```python
from build123d import *

# Parameters (mm, degrees)
BOSS_EXTRUDE1_DEPTH = 3
BOSS_EXTRUDE5_DEPTH = 11.5
SKETCH7_W           = 32.25
SKETCH7_H           = 15
SKETCH7_R           = 3
BOSS_EXTRUDE6_DEPTH = 3.5
FILLET4_R           = 4
FILLET5_R           = 5
FILLET6_SIZE        = 5
FILLET6_SIZE_2      = 15
FILLET7_START       = 5.9999999
FILLET7_DEPTH       = 8.5000001
FILLET7_START_2     = 18.5
FILLET7_2_DEPTH     = 5.5
FILLET8_R           = 7.5
SKETCH9_R           = 1.05
CUT_EXTRUDE2_DEPTH  = 70.629824804
SKETCH10_R          = 1.75
CUT_EXTRUDE3_DEPTH  = 1.5


with BuildPart() as part:
    # Sketch1 → Boss-Extrude1 (new body)
    with BuildSketch(Plane.XY):
        Polygon((7.5, 35), (24.5, 35), (24.5, 56), (-24.5, 56), (-24.5, 35), (-7.5, 35), (-7.5, 0), (7.5, 0), align=None)
    extrude(amount=BOSS_EXTRUDE1_DEPTH)

    # Sketch6 → Boss-Extrude5 (add)
    with BuildSketch(Plane.XY.offset(3)):
        Polygon((-24.5, 35), (-7.5, 35), (-7.5, 0), (7.5, 0), (7.5, 35), (24.5, 35), (24.5, 56), (-24.5, 56), align=None)
        Polygon((-22.5, 37), (-5.5, 37), (-5.5, 2), (5.5, 2), (5.5, 37), (22.5, 37), (22.5, 54), (-22.5, 54), align=None, mode=Mode.SUBTRACT)
    extrude(amount=BOSS_EXTRUDE5_DEPTH)

    # Sketch7 → Boss-Extrude6 (add)
    # profile 1 of 2: a face of its own
    with BuildSketch(Plane(origin=(0, 0, 14.5), x_dir=(-1, 0, 0), z_dir=(0, 0, -1))):
        with Locations((-23.625, 11)):
            Rectangle(SKETCH7_W, SKETCH7_H)
        with Locations((-32.25, 11)):
            Circle(SKETCH7_R, mode=Mode.SUBTRACT)
    # profile 2 of 2: a face of its own
    with BuildSketch(Plane(origin=(0, 0, 14.5), x_dir=(-1, 0, 0), z_dir=(0, 0, -1))):
        with Locations((23.625, 11)):
            Rectangle(SKETCH7_W, SKETCH7_H)
        with Locations(Location((32.25, 11, 0), (0, 0, 180))):
            Circle(SKETCH7_R, mode=Mode.SUBTRACT)
    extrude(amount=BOSS_EXTRUDE6_DEPTH)

    # Fillet4
    fillet4_edges = [part.edges().sort_by_distance(p)[0] for p in [
        (-22.5, 37, 8.75),
        (-5.5, 37, 8.75),
        (-5.5, 2, 8.75),
        (5.5, 2, 8.75),
        (5.5, 37, 8.75),
        (22.5, 37, 8.75),
        (22.5, 54, 8.75),
        (-22.5, 54, 8.75),
    ]]
    fillet(fillet4_edges, radius=FILLET4_R)

    # Fillet5
    fillet5_edges = [part.edges().sort_by_distance(p)[0] for p in [
        (-7.5, 35, 7.25),
        (7.5, 35, 7.25),
        (-7.5, 0, 7.25),
        (7.5, 0, 7.25),
        (0, 0, 0),
        (7.5, 17.5, 0),
        (-7.5, 17.5, 0),
        (-16, 35, 0),
        (16, 35, 0),
        (-24.5, 45.5, 0),
        (24.5, 45.5, 0),
        (0, 56, 0),
        (24.5, 35, 7.25),
        (24.5, 56, 7.25),
        (-24.5, 35, 7.25),
        (-24.5, 56, 7.25),
    ]]
    fillet(fillet5_edges, radius=FILLET5_R)

    # Fillet6
    # a fillet whose section is not a circle: 15, 5 mm, written as the material it adds along each edge
    with BuildSketch(Plane(origin=(-2.5, 5, 11), x_dir=(-1, 0, 0), z_dir=(0, 1, 0))) as fillet6_piece_1_section:
        with BuildLine():
            Bezier((5, -FILLET6_SIZE), (5, 0), (5 + FILLET6_SIZE_2, 0), weights=[1, 0.707106781, 1])
            Line((5 + FILLET6_SIZE_2, 0), (5, 0))
            Line((5, 0), (5, -FILLET6_SIZE))
        make_face()
    fillet6_piece_1 = revolve(axis=Axis((-2.5, 5, 11), (0, 0, 1)), revolution_arc=359.64, mode=Mode.PRIVATE)
    fillet6_piece_1 = split(fillet6_piece_1, bisect_by=Plane(origin=(-2.5, 18.5, 11), z_dir=(0, -1, 0)), keep=Keep.TOP, mode=Mode.PRIVATE)
    fillet6_piece_1 = split(fillet6_piece_1, bisect_by=Plane(origin=(-2.5, 3.5, 11), z_dir=(0, 1, 0)), keep=Keep.TOP, mode=Mode.PRIVATE)
    fillet6_piece_1 = split(fillet6_piece_1, bisect_by=Plane(origin=(-5.5, 5, 11), z_dir=(-1, 0, 0)), keep=Keep.TOP, mode=Mode.PRIVATE)
    add(fillet6_piece_1)
    with BuildSketch(Plane(origin=(-2.5, 5, 11), x_dir=(-1, 0, 0), z_dir=(0, 1, 0))) as fillet6_piece_2_section:
        with BuildLine():
            Bezier((5, -FILLET6_SIZE), (5, 0), (5 + FILLET6_SIZE_2, 0), weights=[1, 0.707106781, 1])
            Line((5 + FILLET6_SIZE_2, 0), (5, 0))
            Line((5, 0), (5, -FILLET6_SIZE))
        make_face()
    fillet6_piece_2 = revolve(axis=Axis((-2.5, 5, 11), (0, 0, 1)), revolution_arc=359.64, mode=Mode.PRIVATE)
    fillet6_piece_2 = split(fillet6_piece_2, bisect_by=Plane(origin=(-2.5, 18.5, 11), z_dir=(0, -1, 0)), keep=Keep.TOP, mode=Mode.PRIVATE)
    fillet6_piece_2 = split(fillet6_piece_2, bisect_by=Plane(origin=(-2.5, 3.5, 11), z_dir=(0, 1, 0)), keep=Keep.TOP, mode=Mode.PRIVATE)
    fillet6_piece_2 = split(fillet6_piece_2, bisect_by=Plane(origin=(5.5, 5, 11), z_dir=(1, 0, 0)), keep=Keep.TOP, mode=Mode.PRIVATE)
    add(fillet6_piece_2)
    with BuildSketch(Plane(origin=(-7.5, 18.5, 11), x_dir=(0, 0, -1), z_dir=(0, -1, 0)), Plane(origin=(7.5, 5, 11), x_dir=(0, 0, -1), z_dir=(0, 1, 0))) as fillet6_piece_3:
        with BuildLine():
            Bezier((FILLET6_SIZE, 0), (0, 0), (0, -FILLET6_SIZE_2), weights=[1, 0.707106781, 1])
            Line((0, -FILLET6_SIZE_2), (0, 0))
            Line((0, 0), (FILLET6_SIZE, 0))
        make_face()
    extrude(amount=13.5)
    with BuildSketch(Plane(origin=(2.5, 5, 11), x_dir=(0.9999802608561371, 0.006283143965559468, 0), z_dir=(0.006283143965559468, -0.9999802608561371, 0))) as fillet6_piece_4_section:
        with BuildLine():
            Bezier((5, -FILLET6_SIZE), (5, 0), (5 + FILLET6_SIZE_2, 0), weights=[1, 0.707106781, 1])
            Line((5 + FILLET6_SIZE_2, 0), (5, 0))
            Line((5, 0), (5, -FILLET6_SIZE))
        make_face()
    fillet6_piece_4 = revolve(axis=Axis((2.5, 5, 11), (0, 0, 1)), revolution_arc=359.64, mode=Mode.PRIVATE)
    fillet6_piece_4 = split(fillet6_piece_4, bisect_by=Plane(origin=(2.5, 18.5, 11), z_dir=(0, -1, 0)), keep=Keep.TOP, mode=Mode.PRIVATE)
    fillet6_piece_4 = split(fillet6_piece_4, bisect_by=Plane(origin=(2.5, 3.5, 11), z_dir=(0, 1, 0)), keep=Keep.TOP, mode=Mode.PRIVATE)
    fillet6_piece_4 = split(fillet6_piece_4, bisect_by=Plane(origin=(5.5, 5, 11), z_dir=(1, 0, 0)), keep=Keep.TOP, mode=Mode.PRIVATE)
    add(fillet6_piece_4)
    with BuildSketch(Plane(origin=(2.5, 5, 11), x_dir=(0.9999802608561371, 0.006283143965559468, 0), z_dir=(0.006283143965559468, -0.9999802608561371, 0))) as fillet6_piece_5_section:
        with BuildLine():
            Bezier((5, -FILLET6_SIZE), (5, 0), (5 + FILLET6_SIZE_2, 0), weights=[1, 0.707106781, 1])
            Line((5 + FILLET6_SIZE_2, 0), (5, 0))
            Line((5, 0), (5, -FILLET6_SIZE))
        make_face()
    fillet6_piece_5 = revolve(axis=Axis((2.5, 5, 11), (0, 0, 1)), revolution_arc=359.64, mode=Mode.PRIVATE)
    fillet6_piece_5 = split(fillet6_piece_5, bisect_by=Plane(origin=(2.5, 18.5, 11), z_dir=(0, -1, 0)), keep=Keep.TOP, mode=Mode.PRIVATE)
    fillet6_piece_5 = split(fillet6_piece_5, bisect_by=Plane(origin=(2.5, 3.5, 11), z_dir=(0, 1, 0)), keep=Keep.TOP, mode=Mode.PRIVATE)
    fillet6_piece_5 = split(fillet6_piece_5, bisect_by=Plane(origin=(-5.5, 5, 11), z_dir=(-1, 0, 0)), keep=Keep.TOP, mode=Mode.PRIVATE)
    add(fillet6_piece_5)

    # Fillet7: read off the stored shape, not the designer's step
    # Fillet7 outline → Fillet7 (add)
    with BuildSketch(Plane.XY.offset(FILLET7_START)):
        with BuildLine():
            Line((-7.5, 18.5), (-7.5, 23.5))
            ThreePointArc((-7.5, 23.5), (-8.964554264, 19.964377926), (-12.500249379, 18.500000006))
            Line((-12.500249379, 18.500000006), (-7.5, 18.5))
        make_face()
        with BuildLine():
            Line((7.5, 18.5), (12.500245622, 18.500000006))
            ThreePointArc((12.500245622, 18.500000006), (8.964552936, 19.964379255), (7.5, 23.5))
            Line((7.5, 23.5), (7.5, 18.5))
        make_face()
    extrude(amount=FILLET7_DEPTH)

    # Fillet7 2 outline → Fillet7 2 (cut)
    with BuildSketch(Plane(origin=(0, 0, 0), x_dir=(1, 0, 0), z_dir=(0, 1, 0)).offset(FILLET7_START_2)):
        with BuildLine():
            Line((-14, -5.9999999), (-14, -10.119735698))
            add(Edge.make_bspline(
                [(-14, -10.119735698), (-7.5, -8.629618531), (-7.5, -6)],
                knots=[0.389274824, 0.389274824, 0.389274824, 1, 1, 1], degree=2, weights=[0.86073517, 0.821122737, 1]))
            Line((-7.5, -6), (-14, -5.9999999))
        make_face()
        with BuildLine():
            add(Edge.make_bspline(
                [(7.5, -6), (7.5, -8.629618531), (14, -10.119735698)],
                knots=[0, 0, 0, 0.610725176, 0.610725176, 0.610725176], degree=2, weights=[1, 0.821122737, 0.86073517]))
            Line((14, -10.119735698), (14, -5.9999999))
            Line((14, -5.9999999), (7.5, -6))
        make_face()
    extrude(amount=FILLET7_2_DEPTH, mode=Mode.SUBTRACT)

    # Fillet8
    fillet8_edges = [part.edges().sort_by_distance(p)[0] for p in [
        (-39.75, 18.5, 12.75),
        (-39.75, 3.5, 12.75),
        (39.75, 18.5, 12.75),
        (39.75, 3.5, 12.75),
    ]]
    fillet(fillet8_edges, radius=FILLET8_R - 0.0001)  # a hair under: the kernel refuses the full size

    # Sketch9 → Cut-Extrude2 (cut, through all)
    with BuildSketch(Plane.XY.offset(3)):
        with Locations((-18.25, 46)):
            Circle(SKETCH9_R)
        with Locations(Location((18.25, 46, 0), (0, 0, 180))):
            Circle(SKETCH9_R)
    extrude(amount=-CUT_EXTRUDE2_DEPTH, mode=Mode.SUBTRACT)

    # Sketch10 → Cut-Extrude3 (cut)
    with BuildSketch(Plane(origin=(0, 0, 0), x_dir=(-1, 0, 0), z_dir=(0, 0, -1))):
        with Locations((-18.25, 46)):
            Circle(SKETCH10_R)
        with Locations((18.25, 46)):
            Circle(SKETCH10_R)
    extrude(amount=-CUT_EXTRUDE3_DEPTH, mode=Mode.SUBTRACT)


solid = part.part
```
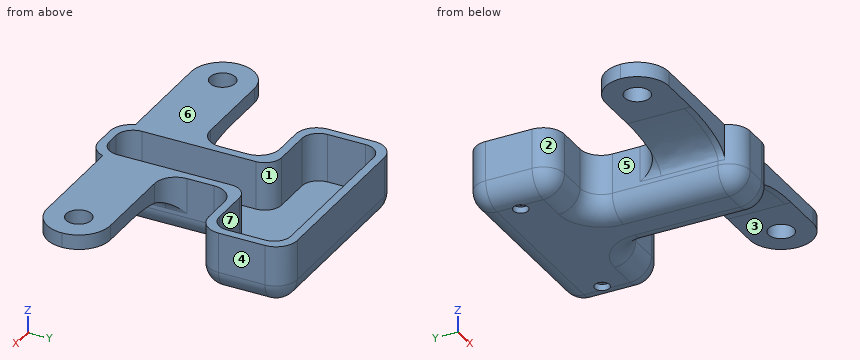
Can you work these out from the model? Positions are in its coordinate system, mm. Face numbers are marked on the shaded views. A direction names the side the tool comes from. Round coordinates to 2 decimals unless told otherwise and drop trailing zeros. Order: outer loops, then holes, each group sorted by start corner. A loop starts at its lowest first (then second) coordinate and runs counter-clockwise, first axis right, second up. Notation, with made-up numbers: (88.25, -1.75) -> (120.25, -1.75) arc R33 ccw to (120.25, 26.25) -> close; hole circle Ø5 at (74, -23). An arc over 180 degrees is marked (long way). Return JSON: item names as keys, results as strings. Group by question number.
1. Will these pins go through, and if not, where does the flat tip stop? pin 1 (4.5 mm diameter, centred on y = 45.5, z = 9.5, fed in from +X); pin 2 (4 mm diameter, centred on x = 22, z = 11, fed in from +Y); pin 3 (2.5 mm diameter, centred on x = -22, z = 11, fed in from +Y).
2. If we section it at A-A, the plane y = 46: Write out the boundary of the cut face in (x, z), then the cut area to 3 significant figures.
3. Which directions (+Z, -Z, +X, -X, +Y, -Y) give clear straight access to the entire face, cutting with the end or side of a thin tool? Please do the marked faces 1, 2 and 3.
4. We'd pull the mould along X, two halves only. Please class the marked faces 4, 5, 6 and 7: released by +X, released by -X, zero draft, split by the parting line, or undercut.
5. If we section it at B-B, the plane x = -33.5: Write out the boundary of the cut face in (y, z), then the cut area to 3 significant figures.
6. I need wall thicknesses on line 1 (Y direction, x = -17.5, z = 5.25); line 2 (X direction, y = 14, z = 6.25); line 3 (Y direction, x = -0.5, z = 9.75). Which ranges of each line are inside material? Lowest first, please. Write a range as [from, to].
Output values:
{
 "1": {"pin 1": "x = 24.5", "pin 2": "y = 55.97", "pin 3": "y = 55.84"},
 "2": {"outline": "(-24.5, 5) arc R5 ccw to (-20, 0.03) -> (-20, 1.5) -> (-19.3, 1.5) -> (-19.3, 3) -> (-22.5, 3) -> (-22.5, 14.5) -> (-24.5, 14.5) -> close; (-17.2, 1.5) -> (-16.5, 1.5) -> (-16.5, 0) -> (16.5, 0) -> (16.5, 1.5) -> (17.2, 1.5) -> (17.2, 3) -> (-17.2, 3) -> close; (19.3, 1.5) -> (20, 1.5) -> (20, 0.03) arc R5 ccw to (24.5, 5) -> (24.5, 14.5) -> (22.5, 14.5) -> (22.5, 3) -> (19.3, 3) -> close", "area": "165 mm²"},
 "3": {"face 1": "+Z", "face 2": "+Z, -Z, -X", "face 3": "-Z, +X, -Y"},
 "4": {"face 4": "released by +X", "face 5": "released by -X", "face 6": "zero draft", "face 7": "undercut"},
 "5": {"outline": "(3.6, 11) -> (8.27, 11) -> (8.27, 14.5) -> (3.6, 14.5) -> close; (13.73, 11) -> (18.4, 11) -> (18.4, 14.5) -> (13.73, 14.5) -> close", "area": "32.7 mm²"},
 "6": {"line 1": "[35, 37], [54, 56]", "line 2": "[-7.52, -5.5], [5.5, 7.52]", "line 3": "[0, 2], [54, 56]"}
}
